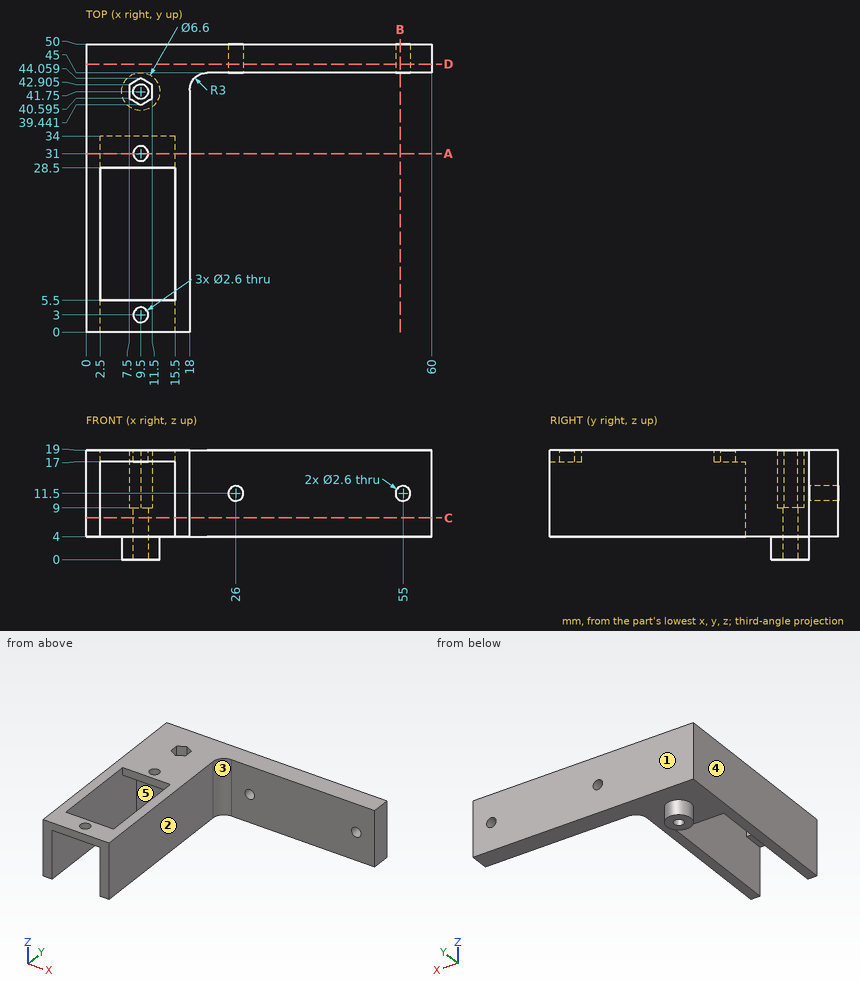
Here's the drawing with two shaded views (mm, measured from the low corner). I have some questions. A direction names the side the tool comes from. Give positions to 0.01 mm unless a question says otherwise; leave off trailing zeros. Order: outer loops, then holes, each group sorted by start corner. A loop starts at its lowest first (then second) coordinate and runs counter-clockwise, first axis right, second up. Notation, with made-up numbers: M 67.25,78.5 L 78.25,78.5 A17 cw 78.25,105.5 Z; hole C 22.25,36 d6. An arc over 180 degrees is marked long. Answer as a JSON object with one key per item and string values. Group by question number.
1) I'm going to push flat-ended pins straight in: pin 1 Ø2 at (x, z) = (55, 11.5) entering from -Y; pin 2 Ø4 at (x, z) = (8.5, 11) entering from -Y; pin 3 Ø1 at (x, z) = (39.5, 11) entering from -Y; pin 4 Ø4 at (x, y) = (9.5, 3) entering from -Z. Where does each tip first touch, or does it pass through?
2) Please list where these lines run through material, in increasing order: L1, parallel to Y at x = 9.5, z = 18.1; L2, parallel to X at y = 27.5, z = 17.5; L3, parallel to Y at x = 9.5, z = 6.75. Write a range as [from, to].
3) Suppose I cut it at D-D, the plane y = 46.5. Write out the boundary of the cut face in (x, z).
4) Suppose I cut it at B-B, the plane x = 54.5. Write out the boundary of the cut face in (y, z), plus the area to 3 significant figures.
5) We'd pull the mould along X, two halves only. Please class the marked faces 3, 4 and 5: pulls with the +X half, pulls with the -X half, needs draft (parallel to the pull), parting line crosses it, or undercut.
6) Suppose I cut it at A-A, the plane y = 31. Write out the boundary of the cut face in (x, z).
7) Suppose I cut it at C-C, the plane z = 7.25. Write out the boundary of the cut face in (x, y).
8) On a 3-axis mill with a long thin cutter (end or side, diameter ignored), from which of +Z, -Z, +X, -X, +Y, -Y can I reach the whole of each face in a straight line? I mean the marked faces 1 and 2. Say none if no direction works.
Results found:
{
 "1": {"pin 1": "through", "pin 2": "y = 34", "pin 3": "y = 45", "pin 4": "z = 17"},
 "2": {"L1": "[0, 1.7], [4.3, 5.5], [28.5, 29.7], [32.3, 39.44], [44.06, 50]", "L2": "[0, 2.5], [15.5, 18]", "L3": "[34, 40.45], [43.05, 50]"},
 "3": {"outline": "M 0,4 L 60,4 L 60,19 L 0,19 Z; hole C 26,11.5 d2.6; hole C 55,11.5 d2.6"},
 "4": {"outline": "M 45,4 L 50,4 L 50,10.3 L 45,10.3 Z; M 45,12.7 L 50,12.7 L 50,19 L 45,19 Z", "area": "63.0 mm²"},
 "5": {"face 3": "pulls with the +X half", "face 4": "pulls with the -X half", "face 5": "undercut"},
 "6": {"outline": "M 0,4 L 2.5,4 L 2.5,17 L 8.2,17 L 8.2,19 L 0,19 Z; M 10.8,17 L 15.5,17 L 15.5,4 L 18,4 L 18,19 L 10.8,19 Z"},
 "7": {"outline": "M 0,0 L 2.5,0 L 2.5,34 L 15.5,34 L 15.5,0 L 18,0 L 18,42 A3 cw 21,45 L 60,45 L 60,50 L 0,50 Z; hole C 9.5,41.75 d2.6"},
 "8": {"face 1": "+Z, -Z, +X, -X, +Y", "face 2": "+Z, -Z, +X, -Y"}
}
